```python
from build123d import *

# Parameters (mm, degrees)
SKETCH_1_R      = 2.5
EXTRUDE_1_DEPTH = 18
SKETCH_2_R      = 2.55
EXTRUDE_2_DEPTH = 7


with BuildPart() as part:
    # 草图1 → 凸台-拉伸1 (new body)
    with BuildSketch(Plane(origin=(0, 0, 0), x_dir=(1, 0, 0), z_dir=(0, 1, 0))):
        Polygon((4.5, 0), (2.25, 3.897114317), (-2.25, 3.897114317), (-4.5, 0), (-2.25, -3.897114317), (2.25, -3.897114317), align=None)
        Circle(SKETCH_1_R, mode=Mode.SUBTRACT)
    extrude(amount=EXTRUDE_1_DEPTH)

    # 草图2 → 凸台-拉伸2 (add)
    with BuildSketch(Plane(origin=(0, 18, 0), x_dir=(1, 0, 0), z_dir=(0, 1, 0))):
        Circle(SKETCH_2_R)
    extrude(amount=EXTRUDE_2_DEPTH)


solid = part.part
```
Input: part model. Units: mm. Frame: model coordinates. A direction names the side the tool comes from. Coordinates: 2 decimals unless noted, no trailing zeros. Loops run counter-clockwise (first coordinate to the right, second up) from the corner with the lowest first, then second, coordinate; pieces in that order, holes last. Notation, with made-up numbers: M 89,66 L 110,66 A27 ccw 110,105 Z; hole C -39,26 d6. An arc over 180 degrees is marked long. Answer in a Markdown table with one row per item.
1. Section A-A, the plane y = 2.5. Output: boundary loops of the cut face in (x, z), then the cut area to 3 significant figures.
Response:
| item | result |
|---|---|
| outline | M -4.5,0 L -2.25,-3.9 L 2.25,-3.9 L 4.5,0 L 2.25,3.9 L -2.25,3.9 Z; hole C 0,0 d5 |
| area | 33.0 mm2 |
2. Section C-C, the plane z = -0.5. Output: boundary loops of the cut face in (x, y), then the cut area to 3 significant figures.
Response:
| item | result |
|---|---|
| outline | M -4.21,0 L -2.45,0 L -2.45,18 L 2.45,18 L 2.45,0 L 4.21,0 L 4.21,18 L 2.5,18 L 2.5,25 L -2.5,25 L -2.5,18 L -4.21,18 Z |
| area | 98.4 mm2 |
3. Draft query along Z for faces 4 (the flat face through (3.39, 8.87, -1.92)), 5 (the cylindrical face through (1.18, 21.45, 2.26)), 6 (the cylindrical face through (-0.54, 8.87, 2.44)), 7 (the flat face through (2, 0, -2)). Return one class per face: pulls with the +Z half, pulls with the -Z half, needs draft (parallel to the pull), parting line crosses it, or undercut.
Response:
| item | result |
|---|---|
| face 4 | pulls with the -Z half |
| face 5 | parting line crosses it |
| face 6 | undercut |
| face 7 | needs draft |
4. First-contact query: pin 1 (1 mm diameter, centred on x = -2.5, y = 7.5, fed in from +Z); pin 2 (3 mm diameter, centred on x = 3, z = -3, fed in from +Y); pin 3 (1 mm diameter, centred on x = -3.5, y = 3.5, fed in from -Z). Flat tips, straight axial feed; report the tip coordinate or a pass-through.
Response:
| item | result |
|---|---|
| pin 1 | stops at z = 3.9 |
| pin 2 | stops at y = 18 |
| pin 3 | stops at z = -2.6 |
5. Reachability of faces 1 (the flat face through (0, 18, 0)), 2 (the flat face through (-3.359, 8.874, -1.976)), 3 (the flat face through (2, 18, -2)) from +Z, -Z, +X, -X, +Y, -Y: full face, straight path, thin tool, end or side. Return the list, or none.
Response:
| item | result |
|---|---|
| face 1 | -Y |
| face 2 | -Z, -X, +Y, -Y |
| face 3 | +Y |
6. Section B-B, the plane x = 0. Output: boundary loops of the cut face in (y, z).
Response:
| item | result |
|---|---|
| outline | M 0,-3.9 L 18,-3.9 L 18,-2.55 L 25,-2.55 L 25,2.55 L 18,2.55 L 18,3.9 L 0,3.9 L 0,2.5 L 18,2.5 L 18,-2.5 L 0,-2.5 Z |
7. Section D-D, the plane y = 21.75. Output: boundary loops of the cut face in (x, z).
Response:
| item | result |
|---|---|
| outline | C 0,0 d5.1 |
8. Material intervals for line 1 (Z direction, x = 0, y = 12); line 2 (X direction, y = 20.75, z = -0.5); line 3 (X direction, y = 4.75, z = 2), sorted ascending.
Response:
| item | result |
|---|---|
| line 1 | z = -3.9 to -2.5, 2.5 to 3.9 |
| line 2 | x = -2.5 to 2.5 |
| line 3 | x = -3.35 to -1.5, 1.5 to 3.35 |
